Could you check a few things on this drawing? It's one solid part, dimensions in mm from its lowest x, y, z. Give positions to 0.01 mm unless a question says otherwise; leave off trailing zeros. Loops run counter-clockwise (first coordinate to the right, second up) from the corner with the lowest first, then second, coordinate; pieces in that order, holes last. Notation, with made-up numbers: M 73,46 L 120,46 A17 ccw 120,77 Z; hole C 35.25,28 d4. An arc over 180 degrees is marked long. Answer as CSV lines item,"result". Start each with the question number.
Item 1: I want a section at D-D on x = 40. List the corners of the cut face in (y, z) for me.
Item 2: If I drill on line 1 along X through (y, z) = (19.25, 25); line 2 along X through (y, z) = (1.65, 25); line 3 along Z through (x, y) = (26.5, 22.5), over which ranges is the centre line in solid material (lowest first)? Write a range as from..to.
Item 3: I want a section at C-C on y = 20. List the corners of the cut face in (x, z) for me.
Item 4: If we mould it in two halves opening along Z, with no side actions, what happens to the marked faces 1, 2 and 3? For each: released by +Z, released by -Z, zero draft, split by the parting line, or undercut.
Item 5: I want a section at A-A on z = 25. List the corners of the cut face in (x, y) for me, plus the area to 3 significant figures.
Item 6: I want a section at B-B on x = 25. List the corners of the cut face in (y, z) for me, plus the area to 3 significant figures.
Item 7: Will these pins go through, and if not, where does the flat tip stop? P1, Ø4, axis at x = 26, z = 24.5, coming from the +Y side; P2, Ø3, axis at y = 27, z = 28, coming from the -X side; P3, Ø10, axis at x = 15.5, y = 11, coming from the +Z side; P4, Ø10, axis at x = 6.5, z = 10, coming from the -Y side.
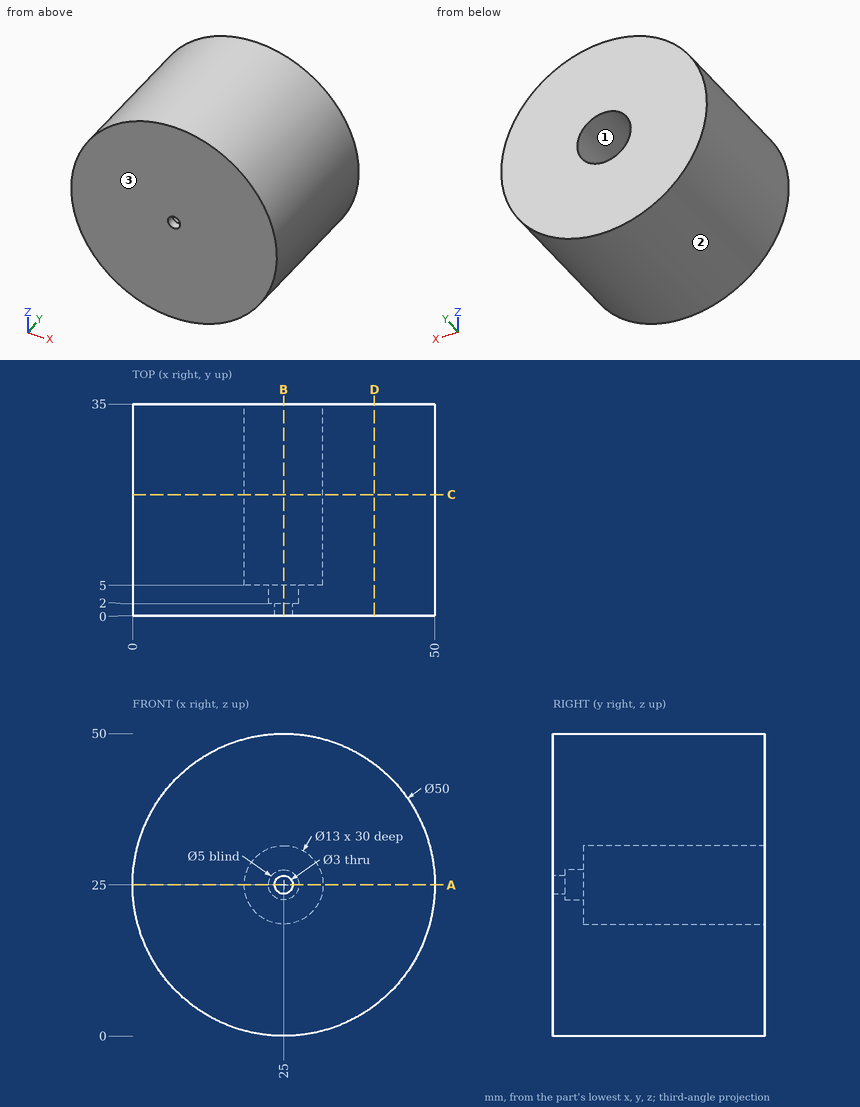
Result:
1,outline,"M 0,5 L 35,5 L 35,45 L 0,45 Z"
2,line 1,"0..18.5, 31.5..50"
2,line 2,"0..23.5, 26.5..50"
2,line 3,"0.05..18.68, 31.32..49.95"
3,outline,"C 25,25 d50; hole C 25,25 d13"
4,face 1,"undercut"
4,face 2,"split by the parting line"
4,face 3,"zero draft"
5,outline,"M 0,0 L 23.5,0 L 23.5,2 L 22.5,2 L 22.5,5 L 18.5,5 L 18.5,35 L 0,35 Z; M 26.5,0 L 50,0 L 50,35 L 31.5,35 L 31.5,5 L 27.5,5 L 27.5,2 L 26.5,2 Z"
5,area,"1,340 mm^2"
6,outline,"M 0,0 L 35,0 L 35,18.5 L 5,18.5 L 5,22.5 L 2,22.5 L 2,23.5 L 0,23.5 Z; M 0,26.5 L 2,26.5 L 2,27.5 L 5,27.5 L 5,31.5 L 35,31.5 L 35,50 L 0,50 Z"
6,area,"1,340 mm^2"
7,P1,"y = 5"
7,P2,"x = 0.05"
7,P3,"z = 49.59"
7,P4,"y = 0"
